Geometry: final body of the model. Coordinates: model frame, mm. A direction names the side the tool comes from. Give positions to 0.01 mm unless a question says otherwise; leave off trailing zeros. Write each loop counter-clockwise with the first axis right and the second up, starting at its lowest first coordinate (ties: lowest second). Pieces come first, ordered by that corner, then holes. Notation, with made-up numbers: (75.25, 46.5) - (133.25, 46.5) arc R31 cw to (133.25, 80.5) - close; hole circle Ø5 at (-7, -20.75). An arc over 180 degrees is marked (long way). Return JSON: item names as keys, results as strings.
from build123d import *

# Parameters (mm, degrees)
EXTRUDE_1_DEPTH              = 23
CUT_EXTRUDE_1_DEPTH          = 84.366660003
CUT_EXTRUDE_1_DEPTH_BACK     = 84.366660003
SKETCH_2_R                   = 3.25
CUT_EXTRUDE_START            = -14
SKETCH_3_W                   = 32.603490834
SKETCH_3_H                   = 14
CUT_EXTRUDE_2_DEPTH          = 70.366660003
FILLET_1_R                   = 10
HOLE_WIZARD_M6_1_D           = 6.6
HOLE_WIZARD_M6_1_CSINK_D     = 13.44
HOLE_WIZARD_M6_1_CSINK_ANGLE = 90
FILLET_2_R                   = 2


with BuildPart() as part:
    # 草图1 → 凸台-拉伸1 (new body)
    with BuildSketch(Plane(origin=(0, 0, 0), x_dir=(1, 0, 0), z_dir=(0, 1, 0))):
        Polygon((-50, 0), (-50, 29), (50, 29), (50, 0), (70, 0), (70, 24), (52, 39), (-52, 39), (-70, 24), (-70, 0), align=None)
    extrude(amount=EXTRUDE_1_DEPTH)

    # 草图2 → 切除-拉伸1 (cut, two sides: drawn at the far end of the back side and taken through both)
    with BuildSketch(Plane.XY.offset(-CUT_EXTRUDE_1_DEPTH_BACK)):
        with Locations(Location((-60, 11.5, 0), (0, 0, 180))):
            Circle(SKETCH_2_R)
        with Locations((60, 11.5)):
            Circle(SKETCH_2_R)
    extrude(amount=CUT_EXTRUDE_1_DEPTH + CUT_EXTRUDE_1_DEPTH_BACK, mode=Mode.SUBTRACT)

    # 草图3 → 切除-拉伸2 (cut, through all)
    with BuildSketch(Plane.XY.offset(CUT_EXTRUDE_START)):
        with Locations((68.801745417, 11.5)):
            Rectangle(SKETCH_3_W, SKETCH_3_H)
        with Locations((-68.801745417, 11.5)):
            Rectangle(SKETCH_3_W, SKETCH_3_H)
    extrude(amount=-CUT_EXTRUDE_2_DEPTH, mode=Mode.SUBTRACT)

    # 圆角1
    fillet_1_edges = [part.edges().sort_by_distance(p)[0] for p in [
        (50, 11.5, -29),
        (-50, 11.5, -29),
    ]]
    fillet(fillet_1_edges, radius=FILLET_1_R)

    # M6 六角凹锥坑螺钉的锥形沉头孔1 (through all)
    with Locations(Plane(origin=(60, 11.5, -14), x_dir=(-1, 0, 0), z_dir=(0, 0, -1))):
        with Locations((0, 0), (120, 0)):
            CounterSinkHole(HOLE_WIZARD_M6_1_D / 2, HOLE_WIZARD_M6_1_CSINK_D / 2, counter_sink_angle=HOLE_WIZARD_M6_1_CSINK_ANGLE)

    # 圆角2
    fillet_2_edges = [part.edges().sort_by_distance(p)[0] for p in [
        (-70, 0, -12),
        (-61, 0, -31.5),
        (0, 0, -39),
        (61, 0, -31.5),
        (70, 0, -12),
        (60, 0, 0),
        (-50, 0, -9.5),
        (-60, 0, 0),
        (60, 23, 0),
        (70, 23, -12),
        (61, 23, -31.5),
        (0, 23, -39),
        (-61, 23, -31.5),
        (-70, 23, -12),
        (-60, 23, 0),
        (-52.5, 18.5, -26.291666667),
        (-52.5, 4.5, -26.291666667),
        (50, 0, -9.5),
        (50, 23, -9.5),
        (0, 0, -29),
        (0, 23, -29),
        (47.071067812, 0, -26.071067812),
        (47.071067812, 23, -26.071067812),
        (-47.071067812, 0, -26.071067812),
        (-50, 23, -9.5),
        (-47.071067812, 23, -26.071067812),
    ]]
    fillet(fillet_2_edges, radius=FILLET_2_R)


solid = part.part
Q1. Section query A-A, the plane z = -7. Return the cut outline in (x, y).
Answer key:
{"outline": "(-70, 2) arc R2 ccw to (-68, 0) - (-52, 0) arc R2 ccw to (-50, 2) - (-50, 21) arc R2 ccw to (-52, 23) - (-68, 23) arc R2 ccw to (-70, 21) - close; (50, 2) arc R2 ccw to (52, 0) - (68, 0) arc R2 ccw to (70, 2) - (70, 21) arc R2 ccw to (68, 23) - (52, 23) arc R2 ccw to (50, 21) - close; hole circle Ø6.6 at (-60, 11.5); hole circle Ø6.6 at (60, 11.5)"}
Q2. Material intervals for probe 1 along X at (y, z) = (11.5, -3.25); probe 2 along X at (y, z) = (6.5, -19); probe 3 along Y at (x, z) = (-59, -29), sorted ascending. Write a range as [from, to].
Answer key:
{"probe 1": "x = [-70, -63.3], [-56.7, -50], [50, 56.7], [63.3, 70]", "probe 2": "x = [-52.5, -50], [50, 52.5]", "probe 3": "y = [0, 4.5], [18.5, 23]"}
Q3. Set-up query: faces 1 (the flat face through (-67, 12, -14)), 2 (the cylindrical face through (-60.761, 0.601, -30.957)), 3 (the flat face through (50, 11, -10)), 4 (the flat face through (59, 4.5, -23)), 5 (the cylindrical face through (60.509, 0.601, -31.167)). Return all of +Z, -Z, +X, -X, +Y, -Y with unobstructed straight access to the full face (end or side cutting, diameter ignored); none if empty.
Answer key:
{"face 1": "-Z, -X", "face 2": "-Z, -X, -Y", "face 3": "+Z, +Y, -Y", "face 4": "-Z, +X", "face 5": "-Z, +X, -Y"}
Q4. Pin query (flat end, axial travel): P1, Ø6, axis at x = 60, y = 11.5, coming from the +Z side (3 decimals); P2, Ø5.5, axis at x = -5.5, y = 15.5, coming from the +Z side; P3, Ø7, axis at x = -57.5, y = 14, coming from the -Z side; P4, Ø5, axis at x = 46, y = 20, coming from the +Z side. Return the tip coordinate at first contact, or that it passes through.
Answer key:
{"P1": "passes through", "P2": "stops at z = -29", "P3": "stops at z = -14", "P4": "stops at z = -24.27"}
Q5. Mould query, pull axis X, two halves, no side actions, for faces 6 (the flat face through (-70, 11, -10)), 7 (the cylindrical face through (57.381, 9.492, -5.216)), 8 (the cylindrical face through (60.49, 22.43, -31.14)). Classes: pulls with the +X half, pulls with the -X half, needs draft (parallel to the pull), parting line crosses it, or undercut.
Answer key:
{"face 6": "pulls with the -X half", "face 7": "undercut", "face 8": "pulls with the +X half"}
Q6. Section query C-C, the plane z = -17.5. Return the cut outline in (x, y), plus the area to 3 significant figures.
Answer key:
{"outline": "(-70, 2) arc R2 ccw to (-68, 0) - (-52, 0) arc R2 ccw to (-50, 2) - (-50, 21) arc R2 ccw to (-52, 23) - (-68, 23) arc R2 ccw to (-70, 21) - (-70, 18.5) - (-54.5, 18.5) arc R2 cw to (-52.5, 16.5) - (-52.5, 6.5) arc R2 cw to (-54.5, 4.5) - (-70, 4.5) - close; (50, 2) arc R2 ccw to (52, 0) - (68, 0) arc R2 ccw to (70, 2) - (70, 4.5) - (52.5, 4.5) - (52.5, 18.5) - (70, 18.5) - (70, 21) arc R2 ccw to (68, 23) - (52, 23) arc R2 ccw to (50, 21) - close", "area": "425 mm^2"}
Q7. Section query B-B, the plane y = 11.5. Return the cut outline in (x, z), plus the area to 3 significant figures.
Answer key:
{"outline": "(-70, -14) - (-66.72, -14) - (-63.3, -10.58) - (-63.3, 0) - (-70, 0) - close; (-56.7, -10.58) - (-53.28, -14) - (-52.5, -14) - (-52.5, -38.58) - (-52, -39) - (52, -39) - (52.5, -38.58) - (52.5, -14) - (53.28, -14) - (56.7, -10.58) - (56.7, 0) - (50, 0) - (50, -19) arc R10 cw to (40, -29) - (-40, -29) arc R10 cw to (-50, -19) - (-50, 0) - (-56.7, 0) - close; (63.3, -10.58) - (66.72, -14) - (70, -14) - (70, 0) - (63.3, 0) - close", "area": "1,520 mm^2"}
Q8. Section query D-D, the plane x = -17. Return the cut outline in (y, z), plus the area to 3 significant figures.
Answer key:
{"outline": "(0, -37) arc R2 ccw to (2, -39) - (21, -39) arc R2 ccw to (23, -37) - (23, -31) arc R2 ccw to (21, -29) - (2, -29) arc R2 ccw to (0, -31) - close", "area": "227 mm^2"}
